from build123d import *

# Parameters (mm, degrees)
SKETCH1_W           = 20
SKETCH1_H           = 30
BOSS_EXTRUDE1_DEPTH = 7
SKETCH2_W           = 30
SKETCH2_H           = 5
CUT_EXTRUDE1_DEPTH  = 2
SKETCH3_W           = 30
SKETCH3_H           = 5
CUT_EXTRUDE2_DEPTH  = 2
SKETCH4_R           = 4
CUT_EXTRUDE3_DEPTH  = 10


with BuildPart() as part:
    # Sketch1 → Boss-Extrude1 (new body)
    with BuildSketch(Plane(origin=(0, 0, 0), x_dir=(1, 0, 0), z_dir=(0, 1, 0))):
        Rectangle(SKETCH1_W, SKETCH1_H)
    extrude(amount=BOSS_EXTRUDE1_DEPTH)

    # Sketch2 → Cut-Extrude1 (cut)
    with BuildSketch(Plane(origin=(10, 0, 0), x_dir=(0, 0, -1), z_dir=(1, 0, 0))):
        with Locations((0, 3.5)):
            Rectangle(SKETCH2_W, SKETCH2_H)
    extrude(amount=-CUT_EXTRUDE1_DEPTH, mode=Mode.SUBTRACT)

    # Sketch3 → Cut-Extrude2 (cut)
    with BuildSketch(Plane.ZY.offset(10)):
        with Locations((0, 3.5)):
            Rectangle(SKETCH3_W, SKETCH3_H)
    extrude(amount=-CUT_EXTRUDE2_DEPTH, mode=Mode.SUBTRACT)

    # Sketch4 → Cut-Extrude3 (cut)
    with BuildSketch(Plane(origin=(0, 7, 0), x_dir=(1, 0, 0), z_dir=(0, 1, 0))):
        Circle(SKETCH4_R)
    extrude(amount=-CUT_EXTRUDE3_DEPTH, mode=Mode.SUBTRACT)


solid = part.part
Input: part model. Units: mm. Frame: model coordinates. A direction names the side the tool comes from. Round coordinates to 2 decimals unless told otherwise and drop trailing zeros. Write each loop counter-clockwise with the first axis right and the second up, starting at its lowest first coordinate (ties: lowest second). Pieces come first, ordered by that corner, then holes.
1) Ray query, L1, parallel to X at y = 5.25, z = 0; L2, parallel to Z at x = 0, y = 4.25; L3, parallel to X at y = 3, z = -9.5. Return the intervals inside material, ascending.
2) Contact query for flat-ended pins moving along their axis: P1, Ø10.5, axis at x = 0, z = 0, coming from the +Y side; P2, Ø2.5, axis at y = 2.5, z = 2.5, coming from the -X side; P3, Ø3, axis at y = 4, z = -5.5, coming from the +X side. Output: stop coordinate, or through.
3) Cut plane D-D (y = 2). Return the cut outline in (x, z), then the cut area to 3 significant figures.
4) Cut plane C-C (z = 11). Return the cut outline in (x, y), then the cut area to 3 significant figures.
5) Cut plane B-B (z = 0). Return the cut outline in (x, y).
6) Reachability of faces 4 (the flat face through (-10, 0.5, 0.2)), 5 (the flat face through (-9, 6, 0)), 6 (the flat face through (8, 4, 0)) from +Z, -Z, +X, -X, +Y, -Y: full face, straight path, thin tool, end or side. Return the list, or none.
7) Cut plane A-A (x = 0). Return the cut outline in (y, z), then the cut area to 3 significant figures.
8) Draft query along Y for faces 1 (the flat face through (10, 6.5, 0.2)), 2 (the flat face through (-2, 0, -4)), 3 (the flat face through (-8, 4, 0)). Return one class per face: pulls with the +Y half, pulls with the -Y half, needs draft (parallel to the pull), parting line crosses it, or undercut.
Geometry says:
1. L1: x = -8 to -4, 4 to 8
1. L2: z = -15 to -4, 4 to 15
1. L3: x = -8 to 8
2. P1: stops at y = 7
2. P2: stops at x = -8
2. P3: stops at x = 8
3. outline: (-8, -15) - (8, -15) - (8, 15) - (-8, 15) - close; hole circle Ø8 at (0, 0)
3. area: 430 mm2
4. outline: (-10, 0) - (10, 0) - (10, 1) - (8, 1) - (8, 6) - (10, 6) - (10, 7) - (-10, 7) - (-10, 6) - (-8, 6) - (-8, 1) - (-10, 1) - close
4. area: 120 mm2
5. outline: (-10, 0) - (-4, 0) - (-4, 7) - (-10, 7) - (-10, 6) - (-8, 6) - (-8, 1) - (-10, 1) - close; (4, 0) - (10, 0) - (10, 1) - (8, 1) - (8, 6) - (10, 6) - (10, 7) - (4, 7) - close
6. face 4: +Z, -Z, -X, +Y, -Y
6. face 5: +Z, -Z, -X
6. face 6: +Z, -Z, +X
7. outline: (0, -15) - (7, -15) - (7, -4) - (0, -4) - close; (0, 4) - (7, 4) - (7, 15) - (0, 15) - close
7. area: 154 mm2
8. face 1: needs draft
8. face 2: pulls with the -Y half
8. face 3: undercut
